The model under review builds one solid part; all positions refer to its coordinate system, in mm. Face numbers are marked on the shaded views. A direction names the side the tool comes from. Coordinates: 2 decimals unless noted, no trailing zeros. Order: outer loops, then holes, each group sorted by start corner. A loop starts at its lowest first (then second) coordinate and runs counter-clockwise, first axis right, second up. Notation, with made-up numbers: (73, 41.25) -> (114, 41.25) arc R20 ccw to (114, 54.25) -> close; hole circle Ø2 at (78.5, -32.75). An arc over 180 degrees is marked (long way). Use one line per item in the form item = value.
from build123d import *

# Parameters (mm, degrees)
F0_W     = 177.8
F0_H     = 38.1
F1_DEPTH = 88.9
F2_W     = 127
F2_H     = 38.1
F3_DEPTH = 38.101
F5_D     = 6.35


with BuildPart() as f1:
    # F0 (on Top) → F1 (new body)
    with BuildSketch(Plane.XY):
        with Locations((88.9, -19.05)):
            Rectangle(F0_W, F0_H)
    extrude(amount=F1_DEPTH)

    # F2 (on face) → F3 (cut, through all)
    with BuildSketch(Plane.XZ.offset(38.1)):
        with Locations((63.5, 19.05)):
            Rectangle(F2_W, F2_H)
    extrude(amount=-F3_DEPTH, mode=Mode.SUBTRACT)

    # F5 (through all)
    with Locations(Plane.XZ.offset(38.1)):
        with Locations((38.1, 63.5), (12.7, 63.5)):
            Hole(F5_D / 2)


solid = f1.part
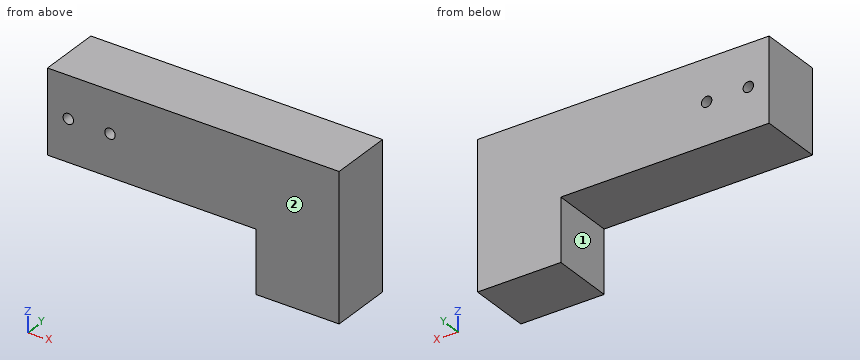
Item 1: To check wall thickness, follow L1, parallel to X at y = -16, z = 63; L2, parallel to Z at x = 12.7, y = -12 (3 decimals); L3, parallel to X at y = -33.5, z = 30.5. State the ranges of each line that lie inside material, in increasing order. Write a range as from..to.
Results found:
L1 = 0..9.56, 15.84..34.96, 41.24..177.8
L2 = 38.1..60.325, 66.675..88.9
L3 = 127..177.8
Item 2: Tool access review of the marked faces 1 and 2: name each direction out of +Z, -Z, +X, -X, +Y, -Y from which nothing blocks a thin tool from reaching the whole face with its end or side.
Results found:
face_1 = -Z, -X, +Y, -Y
face_2 = +Z, -Z, +X, -X, -Y
Item 3: We need section D-D (x = 97.5). Write out the cut boundary in (y, z), plus the area to 3 significant figures.
Results found:
outline = (-38.1, 38.1) -> (0, 38.1) -> (0, 88.9) -> (-38.1, 88.9) -> close
area = 1,940 mm²
Item 4: We need section C-C (z = 63.5). Write out the cut boundary in (x, y) (3 decimals), plus the area to 3 significant figures.
Results found:
outline = (0, -38.1) -> (9.525, -38.1) -> (9.525, 0) -> (0, 0) -> close; (15.875, -38.1) -> (34.925, -38.1) -> (34.925, 0) -> (15.875, 0) -> close; (41.275, -38.1) -> (177.8, -38.1) -> (177.8, 0) -> (41.275, 0) -> close
area = 6,290 mm²
Item 5: We need section A-A (x = 12.7). Write out the cut boundary in (y, z) (3 decimals), plus the area to 3 significant figures.
Results found:
outline = (-38.1, 38.1) -> (0, 38.1) -> (0, 60.325) -> (-38.1, 60.325) -> close; (-38.1, 66.675) -> (0, 66.675) -> (0, 88.9) -> (-38.1, 88.9) -> close
area = 1,690 mm²
Item 6: We need section B-B (y = -33). Write out the cut boundary in (x, z) (3 decimals), plus the area to 3 significant figures.
Results found:
outline = (0, 38.1) -> (127, 38.1) -> (127, 0) -> (177.8, 0) -> (177.8, 88.9) -> (0, 88.9) -> close; hole circle Ø6.35 at (12.7, 63.5); hole circle Ø6.35 at (38.1, 63.5)
area = 10,900 mm²
Item 7: Clearance check with a flat-ended pin moving along its axis: pin 1 (1 mm diameter, centred on x = 25.5, y = -8.5, fed in from -Z). State where the tip first meets the part, or that it passes through.
Results found:
pin_1 = 38.1
